```python
from build123d import *

# Parameters (mm, degrees)
SKETCH1_W           = 88.9
SKETCH1_H           = 76.2
BOSS_EXTRUDE1_DEPTH = 25.4
CUT_EXTRUDE1_DEPTH  = 120.811560377
BOSS_EXTRUDE2_DEPTH = 12.7


with BuildPart() as part:
    # Sketch1 → Boss-Extrude1 (new body)
    with BuildSketch(Plane(origin=(0, 0, 0), x_dir=(1, 0, 0), z_dir=(0, 1, 0))):
        with Locations((44.45, 38.1)):
            Rectangle(SKETCH1_W, SKETCH1_H)
    extrude(amount=BOSS_EXTRUDE1_DEPTH)

    # Sketch2 → Cut-Extrude1 (cut, through all)
    with BuildSketch(Plane(origin=(88.9, 0, 0), x_dir=(0, 0, -1), z_dir=(1, 0, 0))):
        Polygon((76.2, 25.4), (0, 0), (0, 25.4), align=None)
    extrude(amount=-CUT_EXTRUDE1_DEPTH, mode=Mode.SUBTRACT)

    # Sketch3 → Boss-Extrude2 (add)
    with BuildSketch(Plane(origin=(0, 0, 0), x_dir=(1, 0, 0), z_dir=(0, 0.9486832980505139, 0.3162277660168379))):
        Polygon((0, 29.521852568), (2.54, 29.521852568), (2.54, 77.781852568), (86.36, 77.781852568), (86.36, 29.521852568), (88.9, 29.521852568), (88.9, 80.321852568), (0, 80.321852568), align=None)
    extrude(amount=BOSS_EXTRUDE2_DEPTH)


solid = part.part
```
For this review, take the finished solid that the model builds, in its own axes (mm). A direction names the side the tool comes from. Round coordinates to 2 decimals unless told otherwise and drop trailing zeros. Loops run counter-clockwise (first coordinate to the right, second up) from the corner with the lowest first, then second, coordinate; pieces in that order, holes last.
(1) Clearance check with flat-ended pins moving along their axes: P1, Ø8, axis at y = 16.5, z = -19.5, coming from the -X side; P2, Ø3, axis at x = 41, z = -36, coming from the +Y side; P3, Ø2, axis at x = 37.5, z = -8, coming from the +Y side. State where each tip first meets the part, or that it passes through.
Returned:
P1: passes through
P2: stops at y = 12.5
P3: stops at y = 3
(2) Mouldability with a two-part tool opening along X and no side actions: class faces 4 (the flat face through (88.9, 14, -46)), 5 (the flat face through (2.54, 23, -49)), 6 (the flat face through (44, 13, -76.2)) as released by +X, released by -X, zero draft, split by the parting line, or undercut.
Returned:
face 4: released by +X
face 5: undercut
face 6: zero draft
(3) We need section A-A (y = 12.5). Give the boundary of the cut face in (x, z), plus the area to 3 significant figures.
Returned:
outline: (0, -76.2) - (88.9, -76.2) - (88.9, -26.95) - (86.36, -26.95) - (86.36, -37.5) - (2.54, -37.5) - (2.54, -26.95) - (0, -26.95) - close
area: 3,490 mm2
(4) Wall thickness on line 1 along X through (y, z) = (24, -35); line 2 along Y through (x, z) = (40.5, -45); line 3 along Z through (x, y) = (9, 26): over which ranges is each line inside the solid? List them lowest first.
Returned:
line 1: x = 0 to 2.54, 86.36 to 88.9
line 2: y = 0 to 15
line 3: z = -76 to -73.32
(5) We need section C-C (z = -46.5). Give the boundary of the cut face in (x, y).
Returned:
outline: (0, 0) - (88.9, 0) - (88.9, 28.89) - (86.36, 28.89) - (86.36, 15.5) - (2.54, 15.5) - (2.54, 28.89) - (0, 28.89) - close
(6) We need section B-B (x = 22). Give the boundary of the cut face in (y, z), plus the area to 4 significant figures.
Returned:
outline: (0, -76.2) - (25.4, -76.2) - (37.45, -72.18) - (36.65, -69.77) - (24.6, -73.79) - (0, 0) - close
area: 1,000 mm2
(7) Tool access review of faces 1 (the flat face through (87.612, 15.275, -26.027)), 2 (the flat face through (43.86, 30.54, -71.81)), 3 (the flat face through (44.243, 37.188, -71.404)): name each direction out of +Z, -Z, +X, -X, +Y, -Y from which nothing blocks a thin tool from reaching the whole face with its end or side.
Returned:
face 1: +Z, +X, -X
face 2: +Z
face 3: +Z, +X, -X, +Y
(8) We need section D-D (z = -18). Give the boundary of the cut face in (x, y), plus the area to 3 significant figures.
Returned:
outline: (0, 0) - (88.9, 0) - (88.9, 6) - (0, 6) - close
area: 533 mm2
